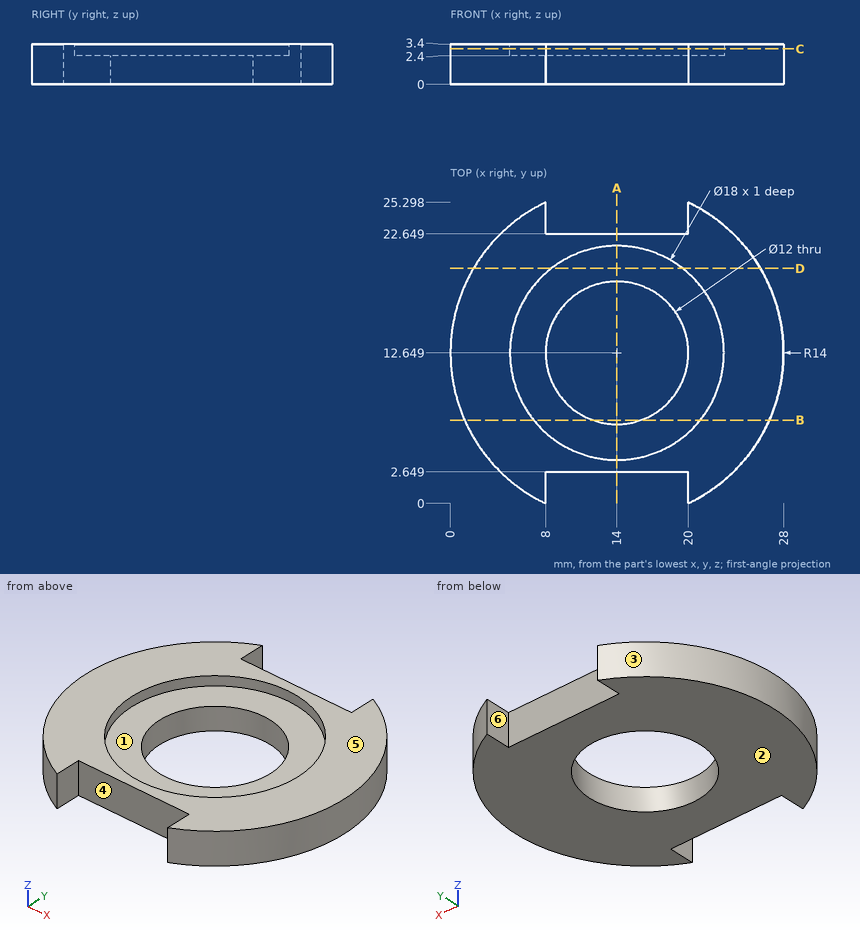
Part print with two shaded views. Sizes in mm from the minimum x, y, z corner. A direction names the side the tool comes from. Round coordinates to 2 decimals unless told otherwise and drop trailing zeros. Loops run counter-clockwise (first coordinate to the right, second up) from the corner with the lowest first, then second, coordinate; pieces in that order, holes last. Notation, with made-up numbers: M -21.5,68 L 14.5,68 A14 cw 14.5,75 Z; hole C 64.25,51.25 d11. An arc over 180 degrees is marked long. Return JSON: item names as keys, results as strings. Group by question number.
(1) Tool access for the marked faces 4, 5 and 6: list every direction of +Z, -Z, +X, -X, +Y, -Y with a clear straight run to the whole face (end or side of a thin tool).
(2) Drop flat-ended pins along their axis: P1, Ø14.5, axis at x = 12.5, y = 17, coming from the +Z side; P2, Ø2, axis at y = 8.5, z = 1, coming from the +X side; P3, Ø2, axis at y = 24, z = 1.5, coming from the +X side; P4, Ø2, axis at y = 24.5, z = 1, coming from the -X side. Give the stop position or say it passes through.
(3) Wall check: probe 1 along Y at (x, z) = (14, 3.05); probe 2 along X at (y, z) = (20.5, 2.55); probe 3 along Y at (x, z) = (16.75, 0.75). Give the ranges that are in metal, low to high. Write a range as [from, to].
(4) Saw through at A-A, the plane x = 14. List the corners of the cut face in (y, z), and give its area (3 significant figures).
(5) Mould opens along Y. For the marked faces 1, 2 and 3 say: +Y half, -Y half, draft (parallel to the pull), parting line (faces both ways), or undercut.
(6) Saw through at C-C, the plane z = 3. List the corners of the cut face in (x, y), and give its area (3 significant figures).
(7) Saw through at B-B, the plane y = 7. List the corners of the cut face in (x, z), and give its area (3 significant figures).
(8) Saw through at D-D, the plane y = 19.75. List the corners of the cut face in (x, z).
Answer list:
{
 "1": {"face 4": "+Z, -Z, -Y", "face 5": "+Z, +X, -X, +Y, -Y", "face 6": "+Z, -Z, +Y"},
 "2": {"P1": "z = 3.4", "P2": "x = 27.64", "P3": "x = 23.43", "P4": "x = 5.15"},
 "3": {"probe 1": "[2.65, 3.65], [21.65, 22.65]", "probe 2": "[2.41, 9.6], [18.4, 25.59]", "probe 3": "[2.65, 7.32], [17.98, 22.65]"},
 "4": {"outline": "M 2.65,0 L 6.65,0 L 6.65,2.4 L 3.65,2.4 L 3.65,3.4 L 2.65,3.4 Z; M 18.65,0 L 22.65,0 L 22.65,3.4 L 21.65,3.4 L 21.65,2.4 L 18.65,2.4 Z", "area": "21.2 mm2"},
 "5": {"face 1": "undercut", "face 2": "draft", "face 3": "parting line"},
 "6": {"outline": "M 8,0 L 8,2.65 L 20,2.65 L 20,0 A14 ccw 20,25.3 L 20,22.65 L 8,22.65 L 8,25.3 A14 ccw Z; hole C 14,12.65 d18", "area": "276 mm2"},
 "7": {"outline": "M 1.19,0 L 11.98,0 L 11.98,2.4 L 6.99,2.4 L 6.99,3.4 L 1.19,3.4 Z; M 16.02,0 L 26.81,0 L 26.81,3.4 L 21.01,3.4 L 21.01,2.4 L 16.02,2.4 Z", "area": "63.4 mm2"},
 "8": {"outline": "M 1.93,0 L 26.07,0 L 26.07,3.4 L 19.53,3.4 L 19.53,2.4 L 8.47,2.4 L 8.47,3.4 L 1.93,3.4 Z"}
}
